Part model, mm, in its own coordinate system. A direction names the side the tool comes from. Round coordinates to 2 decimals unless told otherwise and drop trailing zeros. Write each loop counter-clockwise with the first axis right and the second up, starting at its lowest first coordinate (ties: lowest second). Pieces come first, ordered by that corner, then holes.
```python
from build123d import *

# Parameters (mm, degrees)
SKETCH1_R               = 42.0875
BOSS_EXTRUDE1_DEPTH     = 16.5
SKETCH2_R               = 38.4875
CUT_EXTRUDE1_DEPTH      = 8.5
SKETCH3_R               = 34.4875
CUT_EXTRUDE2_DEPTH      = 5
SKETCH5_R               = 3.2
CUT_EXTRUDE4_DEPTH      = 1
CUT_EXTRUDE4_DEPTH_BACK = 17.5
CUT_EXTRUDE3_START      = -4
SKETCH4_R               = 1.5
CUT_EXTRUDE3_DEPTH      = 18.5
CIRPATTERN1_COUNT       = 4


with BuildPart() as part:
    # Sketch1 → Boss-Extrude1 (new body)
    with BuildSketch(Plane.XY.offset(-8)):
        Circle(SKETCH1_R)
    extrude(amount=BOSS_EXTRUDE1_DEPTH)

    # Sketch2 → Cut-Extrude1 (cut)
    with BuildSketch(Plane(origin=(0, 0, -8), x_dir=(-1, 0, 0), z_dir=(0, 0, -1))):
        Circle(SKETCH2_R)
    extrude(amount=-CUT_EXTRUDE1_DEPTH, mode=Mode.SUBTRACT)

    # Sketch3 → Cut-Extrude2 (cut)
    with BuildSketch(Plane(origin=(0, 0, 0.5), x_dir=(-1, 0, 0), z_dir=(0, 0, -1))):
        Circle(SKETCH3_R)
    extrude(amount=-CUT_EXTRUDE2_DEPTH, mode=Mode.SUBTRACT)

    # Sketch5 → Cut-Extrude4 (cut, two sides)
    with BuildSketch(Plane.XY.offset(8.5)) as cut_extrude4_sk:
        with Locations((-8.061017306, 8.061017306)):
            Circle(SKETCH5_R)
    extrude(amount=CUT_EXTRUDE4_DEPTH, mode=Mode.SUBTRACT)
    extrude(cut_extrude4_sk.sketch, amount=-CUT_EXTRUDE4_DEPTH_BACK, mode=Mode.SUBTRACT)

    # Sketch4 → Cut-Extrude3 (cut)
    with BuildSketch(Plane(origin=(0, 0, 5.5), x_dir=(-1, 0, 0), z_dir=(0, 0, -1)).offset(CUT_EXTRUDE3_START)):
        with Locations((-16.5, 0)):
            Circle(SKETCH4_R)
    cut_extrude3 = extrude(amount=CUT_EXTRUDE3_DEPTH, mode=Mode.SUBTRACT)

    # CirPattern1: Cut-Extrude3 ×4 about axis
    cirpattern1_axis = Axis((0, 0, 0), (0, 0, 1))
    for i in range(1, CIRPATTERN1_COUNT):
        add(cut_extrude3.rotate(cirpattern1_axis, i * 360 / CIRPATTERN1_COUNT), mode=Mode.SUBTRACT)


solid = part.part
```
Q1. Cut at C-C on z = -6.25. Write the cut outline in (x, y) (1 decimal), plus the area to 3 significant figures.
Values follow:
outline: circle Ø84.2 at (0, 0); hole circle Ø77 at (0, 0)
area: 911 mm2
Q2. Cut at A-A on x = 0. Write the cut outline in (y, z).
Values follow:
outline: (-42.09, -8) - (-38.49, -8) - (-38.49, 0.5) - (-34.49, 0.5) - (-34.49, 5.5) - (-18, 5.5) - (-18, 8.5) - (-42.09, 8.5) - close; (-15, 5.5) - (15, 5.5) - (15, 8.5) - (-15, 8.5) - close; (18, 5.5) - (34.49, 5.5) - (34.49, 0.5) - (38.49, 0.5) - (38.49, -8) - (42.09, -8) - (42.09, 8.5) - (18, 8.5) - close
Q3. Mould opens along X. For faces 3 (the cylindrical face through (40.144, 12.642, 0.134)), 4 (the cylindrical face through (-10.42, 10.224, 7.021)), 5 (the flat face through (19, -34, -8)) say: +X half, -X half, draft (parallel to the pull), parting line (faces both ways), or undercut.
Values follow:
face 3: parting line
face 4: undercut
face 5: draft
Q4. Drop flat-ended pins along their axis: pin 1 (3 mm diameter, centred on y = 15.5, z = 0.5, fed in from -X); pin 2 (1.8 mm diameter, centred on x = 0, y = -16.5, fed in from +Z); pin 3 (6 mm diameter, centred on x = -14.5, y = 13.5, fed in from -Z); pin 4 (3 mm diameter, centred on y = -32.5, z = 3, fed in from -X). Give the stop position or say it passes through.
Values follow:
pin 1: stops at x = -39.69
pin 2: passes through
pin 3: stops at z = 5.5
pin 4: stops at x = -28.47
Q5. Which spindle directions (+Z, -Z, +X, -X, +Y, -Y) get a long thin tool onto all of the face, cutting with end or side? Do faces 1 (the flat face through (0, 0, 5.5)), 2 (the flat face through (-1, 1, 8.5)). Say none if no direction does.
Values follow:
face 1: -Z
face 2: +Z, +X, -X, +Y, -Y
Q6. Wall check: L1, parallel to X at y = -1, z = 7.5; L2, parallel to Y at x = 0, z = 4.4; L3, parallel to Y at x = 0.5, z = -6.5. Give the ranges that are in metal, low to high.
Values follow:
L1: x = -42.08 to -17.62, -15.38 to 15.38, 17.62 to 42.08
L2: y = -42.09 to -34.49, 34.49 to 42.09
L3: y = -42.08 to -38.48, 38.48 to 42.08
Q7. Cut at B-B on y = 16.5. Write the cut outline in (x, z), plus the area to 3 significant figures.
Values follow:
outline: (-38.72, -8) - (-34.77, -8) - (-34.77, 0.5) - (-30.28, 0.5) - (-30.28, 5.5) - (-1.5, 5.5) - (-1.5, 8.5) - (-38.72, 8.5) - close; (1.5, 5.5) - (30.28, 5.5) - (30.28, 0.5) - (34.77, 0.5) - (34.77, -8) - (38.72, -8) - (38.72, 8.5) - (1.5, 8.5) - close
area: 375 mm2
